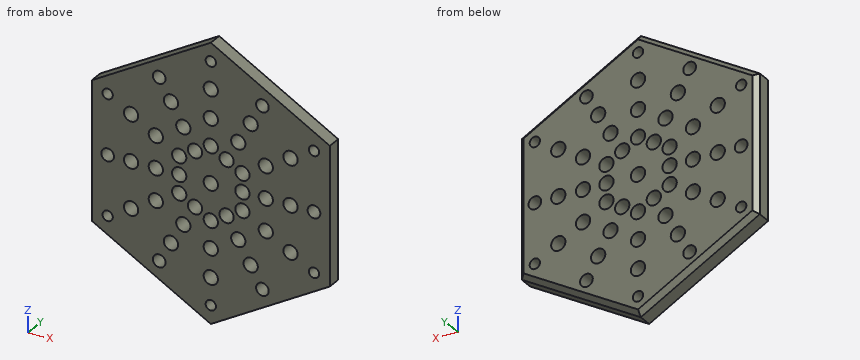
```python
from build123d import *

# Parameters (mm, degrees)
EXTRUDE_2_DEPTH       = 12
CHAMFER_1_SIZE        = 3
F_6_0MM_1_D           = 6.5
F_8_0MM_1_D           = 8
F_6_0MM_2_D           = 9
F_6_0MM_2_ON_FACE_2_D = 9
F_6_0MM_3_D           = 9


with BuildPart() as part:
    # 草圖2 → 填料-伸長2 (new body)
    with BuildSketch(Plane(origin=(0, 0, 0), x_dir=(1, 0, 0), z_dir=(0, 1, 0))):
        Polygon((0, 86.602540378), (-75, 43.301270189), (-75, -43.301270189), (0, -86.602540378), (75, -43.301270189), (75, 43.301270189), align=None)
    extrude(amount=EXTRUDE_2_DEPTH)

    # 導角1
    chamfer_1_edges = [part.edges().sort_by_distance(p)[0] for p in [
        (-75, 12, 0),
        (-37.5, 12, 64.951905284),
        (37.5, 12, 64.951905284),
        (75, 12, 0),
        (37.5, 12, -64.951905284),
        (-37.5, 12, -64.951905284),
    ]]
    chamfer(chamfer_1_edges, length=CHAMFER_1_SIZE)

    # Ø6.0mm 定位孔1 (through all)
    with Locations(Plane(origin=(-65, 12, 37.527767497), x_dir=(0, 0, 1), z_dir=(0, 1, 0))):
        with Locations((0, 0), (-75.055534994, 0), (-112.583302492, 65), (-75.055534994, 130), (37.527767498, 65), (0, 130)):
            Hole(F_6_0MM_1_D / 2)

    # Ø8.0mm 定位孔1 (through all)
    with Locations(Plane(origin=(-65, 12, 0), x_dir=(0, 0, 1), z_dir=(0, 1, 0))):
        with Locations((0, 0), (56.5, 32.5), (56.5, 97.5), (-56.5, 97.5), (-56.5, 32.5), (0, 130)):
            Hole(F_8_0MM_1_D / 2)

    # Ø6.0mm 定位孔2 (through all)
    with Locations(Plane(origin=(-50.229473419, 12, -29), x_dir=(0, 0, 1), z_dir=(0, 1, 0))):
        with Locations((0, 0), (-14.5, 25.114736709), (-29, 50.229473419), (0, 100.458946838), (29, 100.458946838), (72.5, 75.344210129), (87, 50.229473419), (72.5, 25.114736709), (58, 0), (29, 0), (-11, 50.229473419), (9, 84.87048957), (-1, 67.549981495), (-1, 32.908965343), (9, 15.588457268), (17.5, 30.310889132), (11.75, 40.270181275), (6, 50.229473419), (11.75, 60.188765563), (17.5, 70.148057706), (29, 70.148057706), (46.25, 60.188765563), (52, 50.229473419), (46.25, 40.270181275), (40.5, 30.310889132), (49, 15.588457268), (29, 15.588457268), (59, 32.908965343), (69, 50.229473419), (59, 67.549981495), (49, 84.87048957), (29, 84.87048957), (29, 50.229473419)):
            Hole(F_6_0MM_2_D / 2)

    # Ø6.0mm 定位孔2 on face 2 (through all)
    with Locations(Plane(origin=(0, 0, 0), x_dir=(0, 0, -1), z_dir=(0, -1, 0))):
        with Locations((0, 0)):
            Hole(F_6_0MM_2_ON_FACE_2_D / 2)

    # Ø6.0mm 定位孔3 (through all)
    with Locations(Plane(origin=(25.11473671, 12, -43.5), x_dir=(0, 0, 1), z_dir=(0, 1, 0))):
        with Locations((0, 0), (72.5, 25.114736709), (55, -5.196152423), (43.5, -45.033320997)):
            Hole(F_6_0MM_3_D / 2)


solid = part.part
```
The model under review builds one solid part; all positions refer to its coordinate system, in mm. Coordinates: 2 decimals unless noted, no trailing zeros. Write each loop counter-clockwise with the first axis right and the second up, starting at its lowest first coordinate (ties: lowest second). Pieces come first, ordered by that corner, then holes. Notation, with made-up numbers: (39, 63.5) - (83, 63.5) arc R11 ccw to (83, 70.5) - close; hole circle Ø6 at (10.25, 58.5). An arc over 180 degrees is marked (long way). Answer in a Markdown table with one row per item. Add a question column.
Q1. Clearance check with flat-ended pins moving along their axes: pin 1 (4 mm diameter, centred on x = -56.5, z = 54.5, fed in from +Y); pin 2 (6 mm diameter, centred on x = -65, z = 37.53, fed in from -Y); pin 3 (4 mm diameter, centred on x = -2.5, y = 6.5, fed in from -Z); pin 4 (14.5 mm diameter, centred on x = -19.92, z = -11.5, fed in from +Y). State where each tip first meets the part, or that it passes through.
Q2. Consider section A-A on z = -58. Give the boundary of the cut face in (x, y), then the cut area to 3 significant figures.
Q3. Consider section C-C on z = 0. Give the number of separate pieces and of enclosed holes in the cut face, then the cut area to 3 significant figures.
Q4. Consider section B-B on x = -32.5. Give the boundary of the cut face in (y, z), then the cut area to 3 significant figures.
Q5. To check wall thickness, follow line 1 along X through (y, z) = (4, -11.5); line 2 along X through (y, z) = (2.75, -29); line 3 along X through (y, z) = (8.5, 45). State the ranges of each line that lie inside material, in increasing order. Write a range as from..to.
Answers below:
| question | item | result |
|---|---|---|
| 1 | pin 1 | y = 10.55 |
| 1 | pin 2 | through |
| 1 | pin 3 | z = -86.31 |
| 1 | pin 4 | y = 12 |
| 2 | outline | (-49.54, 0) - (-36.21, 0) - (-36.21, 12) - (-43.54, 12) - (-49.54, 9) - close; (-28.79, 0) - (-4.5, 0) - (-4.5, 12) - (-28.79, 12) - close; (4.5, 0) - (28.79, 0) - (28.79, 12) - (4.5, 12) - close; (36.21, 0) - (49.54, 0) - (49.54, 9) - (43.54, 12) - (36.21, 12) - close |
| 2 | area | 885 mm² |
| 3 | separate pieces | 10 |
| 3 | enclosed holes | 0 |
| 3 | area | 843 mm² |
| 4 | outline | (0, -67.84) - (9, -67.84) - (12, -64.37) - (12, -60.5) - (0, -60.5) - close; (0, -52.5) - (12, -52.5) - (12, -23.96) - (0, -23.96) - close; (0, -16.04) - (12, -16.04) - (12, -3.96) - (0, -3.96) - close; (0, 3.96) - (12, 3.96) - (12, 16.04) - (0, 16.04) - close; (0, 23.96) - (12, 23.96) - (12, 52.5) - (0, 52.5) - close; (0, 60.5) - (12, 60.5) - (12, 64.37) - (9, 67.84) - (0, 67.84) - close |
| 4 | area | 1,140 mm² |
| 5 | line 1 | -75..-24.42, -15.42..15.42, 24.42..75 |
| 5 | line 2 | -75..-54.73, -45.73..-21.71, -12.93..12.93, 21.71..45.73, 54.73..75 |
| 5 | line 3 | -72.06..-29.36, -20.87..20.87, 29.36..72.06 |
